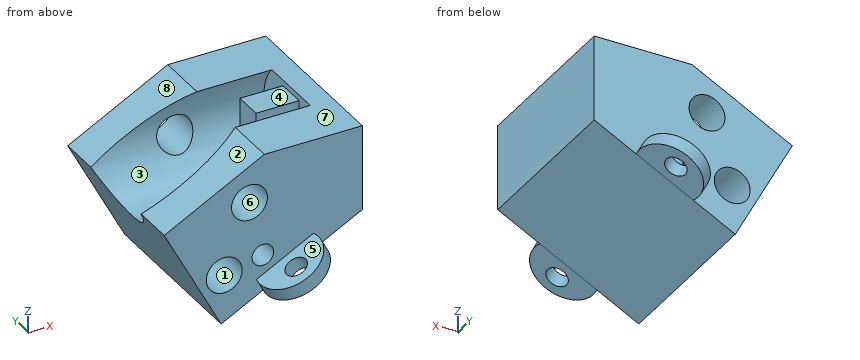
```python
from build123d import *

# Parameters (mm, degrees)
F0_W      = 50.8
F0_H      = 38.1
F1_DEPTH  = 50.8
F3_R      = 10.7442
F4_DEPTH  = 40.64
F5_DEPTH  = 45.72
F7_DEPTH  = 38.101
F9_W      = 6.35
F9_H      = 12.7
F10_DEPTH = 9.525
F11_DEPTH = 38.101
F13_DEPTH = 38.101
F20_R     = 2.38125
F20_R_2   = 3.96875
F20_R_3   = 3.9751
F21_DEPTH = 38.101
F22_DEPTH = 3.175
F23_R     = 2.3876
F24_DEPTH = 3.175


# Not quite as in the source:
# - a feature names something its author has since deleted; it is built from what else it names


with BuildPart() as f1:
    # F0 (on Top) → F1 (new body)
    with BuildSketch(Plane.XY):
        with Locations((25.4, -19.05)):
            Rectangle(F0_W, F0_H)
    extrude(amount=F1_DEPTH)

    # F3 (on face) → F4 (cut)
    with BuildSketch(Plane(origin=(0, 0, 0), x_dir=(0, -1, 0), z_dir=(-1, 0, 0))):
        with Locations((19.05, 43.18)):
            Circle(F3_R)
    extrude(amount=-F4_DEPTH, mode=Mode.SUBTRACT)

    # F3 (on face) → F5 (cut)
    with BuildSketch(Plane(origin=(0, 0, 0), x_dir=(0, -1, 0), z_dir=(-1, 0, 0))):
        with Locations((19.05, 43.18)):
            Circle(F3_R)
    extrude(amount=-F5_DEPTH, mode=Mode.SUBTRACT)

    # F6 (on face) → F7 (cut, through all)
    with BuildSketch(Plane.XZ.offset(38.1)):
        Polygon((-5.2975248545, 32.5760431588), (29.6258907765, 51.0742887855), (29.3069556355, 56.4961917698), (-5.2975248545, 56.4961917698), align=None)
    extrude(amount=-F7_DEPTH, mode=Mode.SUBTRACT)

    # F9 (on face) → F10 (join)
    with BuildSketch(Plane(origin=(45.72, 0, 0), x_dir=(0, -1, 0), z_dir=(-1, 0, 0))):
        with Locations((19.05, 43.18)):
            Rectangle(F9_W, F9_H)
    extrude(amount=F10_DEPTH)

    # F8 (on face) → F11 (cut, through all)
    with BuildSketch(Plane.XZ.offset(38.1)):
        Polygon((12.6081767879, 11.5786670478), (0, 35.3820377673), (-3.8052792661, 35.2523848414), (-3.8052792661, -3.7349041086), (52.9321556466, -3.7349041086), (52.9321556466, 32.9374846805), align=None)
    extrude(amount=-F11_DEPTH, mode=Mode.SUBTRACT)

    # F12 (on face) → F13 (cut, through all)
    with BuildSketch(Plane.XZ.offset(38.1)):
        Polygon((21.0712682456, 12.4185690656), (5.5156808657, 41.7864482914), (-6.4950456949, 35.4714418711), (9.0799157449, 6.0669857527), align=None)
    extrude(amount=-F13_DEPTH, mode=Mode.SUBTRACT)


with BuildPart() as f1_1:
    # F14: moved
    add(f1.part.moved(Location((12.8, 76.1, -11.5))))


with BuildPart() as f1_2:
    # F16: moved
    add(f1_1.part.moved(Location((-7.9, 0, 0))))


with BuildPart() as f1_3:
    # F17: moved
    add(f1_2.part.moved(Location((1.3, 0, -3.7))))


with BuildPart() as f1_4:
    # F18: moved
    add(f1_3.part.moved(Location((0.5, 0, -3.8))))


with BuildPart() as f1_5:
    # F19: moved
    add(f1_4.part.moved(Location((-1.016, 0, 4.064))))

    # F20 (on face) → F21 (cut, through all)
    with BuildSketch(Plane(origin=(0, 76.1, 0), x_dir=(-1, 0, 0), z_dir=(0, 1, 0))):
        with Locations((-34.4707481563, 13.2179586217)):
            Circle(F20_R)
        with Locations((-25.9255170822, 11.1699821427)):
            Circle(F20_R_2)
        with Locations((-31.5185599029, 25.9363166988)):
            Circle(F20_R_3)
    extrude(amount=-F21_DEPTH, mode=Mode.SUBTRACT)

    # F22 (add): a face of the model
    f22_faces = [f1_5.faces().sort_by_distance(p)[0] for p in [
        (40.8662395369, 57.05, 8.5997036085),
    ]]
    extrude(f22_faces, amount=-F22_DEPTH)

    # F23 (on face) → F24 (join)
    with BuildSketch(Plane(origin=(5.3963751445, 0, -10.1879851676), x_dir=(0.8836897656, 0, 0.4680730692), z_dir=(0.4680730692, 0, -0.8836897656))):
        with BuildLine():
            Line((32.9755673007, -38), (47.2757673007, -38))
            ThreePointArc((47.2757673007, -38), (40.1256673007, -29.0169325565), (32.9755673007, -38))
        make_face()
        with Locations((40.1383673007, -33.5931)):
            Circle(F23_R, mode=Mode.SUBTRACT)
        with BuildLine():
            ThreePointArc((32.9755673007, -76.1), (40.1256673007, -85.0830674435), (47.2757673007, -76.1))
            Line((47.2757673007, -76.1), (32.9755673007, -76.1))
        make_face()
        with Locations((40.1383673007, -80.5069)):
            Circle(F23_R, mode=Mode.SUBTRACT)
    extrude(amount=-F24_DEPTH)


solid = f1_5.part
```
Verification items for the finished model (mm, model axes). Face numbers are marked on the shaded views. A direction names the side the tool comes from. Coordinates: 2 decimals unless noted, no trailing zeros. Write each loop counter-clockwise with the first axis right and the second up, starting at its lowest first coordinate (ties: lowest second). Pieces come first, ordered by that corner, then holes. Notation, with made-up numbers: (25, -38.75) - (72, -38.75) arc R26 ccw to (72, -3.75) - close; hole circle Ø6 at (46, 8.5). An arc over 180 degrees is marked (long way). Write item = value, one per line.
Q1. Cross-section at C-C (z = 32.5). Enter the section's corners in (x, y) (3 decimals).
Answer:
outline = (28.441, 38) - (56.484, 38) - (56.484, 76.1) - (28.441, 76.1) - (28.441, 66.915) - (51.404, 66.915) - (51.404, 60.225) - (41.879, 60.225) - (41.879, 53.875) - (51.404, 53.875) - (51.404, 47.185) - (28.441, 47.185) - close
Q2. Cross-section at D-D (x = 17.5). Enter the section's corners in (y, z).
Answer:
outline = (38, 14.96) - (76.1, 14.96) - (76.1, 26.7) - (67.68, 26.7) arc R10.74 cw to (46.42, 26.7) - (38, 26.7) - close
Q3. Material ranges on L1, parallel to Y at x = 51, z = 24 (3 decimals); L2, parallel to X at y = 42, z = 28; L3, parallel to X at y = 40.5, z = 9, recorded low to high. Write a range as from..to.
Answer:
L1 = 38..47.18, 53.875..60.225, 66.92..76.1
L2 = 19.95..28.12, 34.92..56.48
L3 = 20.65..22.6, 29.25..41.62
Q4. Access from +Z, -Z, +X, -X, +Y, -Y to the whole of each face (thin tool, end or side, straight path). Record for the marked faces 1, 2, 3, 4 and 5.
Answer:
face_1 = +Y, -Y
face_2 = +Z, -X, +Y, -Y
face_3 = -X
face_4 = +Z, -X
face_5 = +Z, -X, -Y
Q5. Cross-section at B-B (x = 26.5). Enter the section's corners in (y, z), plus the area to 3 significant figures.
Answer:
outline = (38, 0.99) - (76.1, 0.99) - (76.1, 7.24) - (38, 7.24) - close; (38, 15.1) - (76.1, 15.1) - (76.1, 31.47) - (67.3, 31.47) arc R10.74 cw (long way) to (46.8, 31.47) - (38, 31.47) - close
area = 612 mm²
Q6. Go/stop test with flat-tipped pins: pin 1 Ø12.5 at (x, z) = (25.93, 11.17) entering from +Y; pin 2 Ø18 at (x, z) = (30, 18) entering from -Y; pin 3 Ø1.5 at (y, z) = (35.5, 15.5) entering from +X; pin 4 Ø4.5 at (x, z) = (34.47, 13.22) entering from -Y. Record where each tip stops, or that it passes through.
Answer:
pin_1 = 76.1
pin_2 = 38
pin_3 = 45.85
pin_4 = through
Q7. Cross-section at A-A (y = 57.05). Enter the section's corners in (x, z).
Answer:
outline = (16.15, 17.5) - (25.25, 0.33) - (56.48, 16.87) - (56.48, 35.86) - (51.4, 35.86) - (51.4, 34.59) - (41.88, 34.59) - (41.88, 21.89) - (51.4, 21.89) - (51.4, 17.77) - (50.89, 17.5) - close; hole circle Ø7.94 at (25.93, 11.17); hole circle Ø4.76 at (34.47, 13.22)
Q8. Mould release check, pull along X, two halves, no side actions. Record for the marked faces 6, 7 and 8: released by +X, released by -X, zero draft, split by the parting line, or undercut.
Answer:
face_6 = undercut
face_7 = zero draft
face_8 = released by -X
